Input: dimensioned drawing with shaded views. Units: mm. Origin: part minimum x, y, z. A direction names the side the tool comes from. Coordinates: 2 decimals unless noted, no trailing zeros. Order: outer loops, then holes, each group sorted by start corner. A loop starts at its lowest first (then second) coordinate and runs counter-clockwise, first axis right, second up.
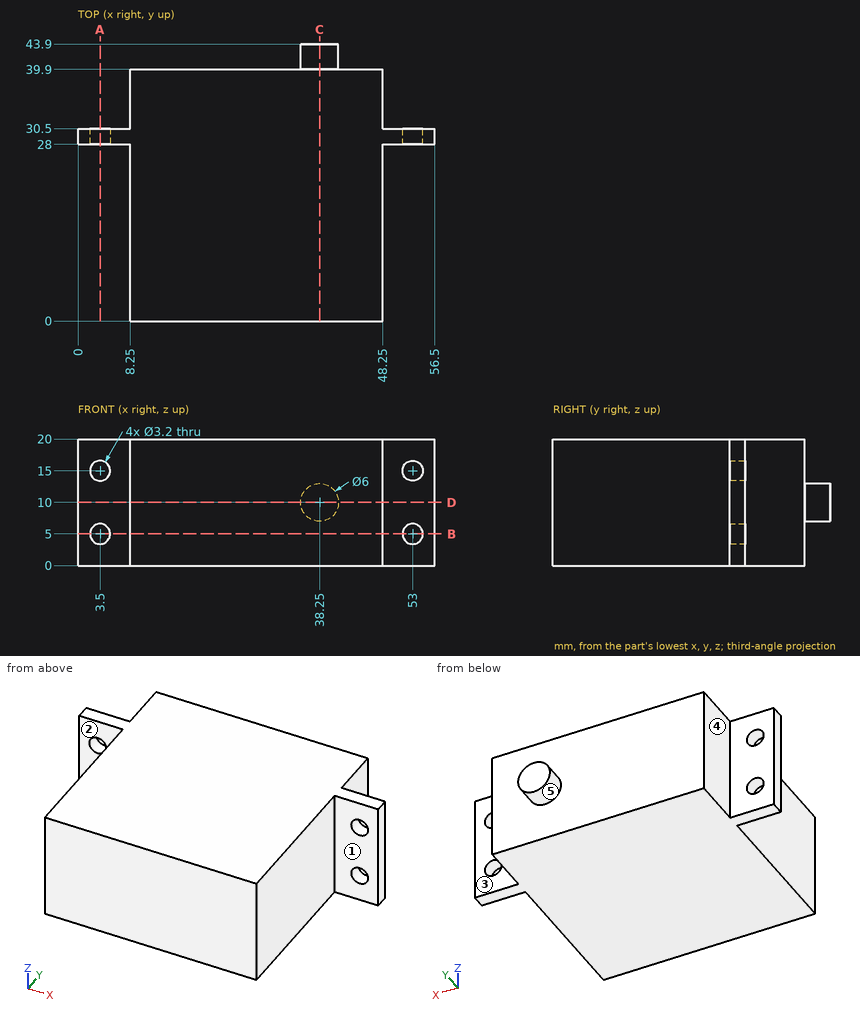
1. Section query D-D, the plane z = 10. Output: boundary loops of the cut face in (x, y), plus the area to 3 significant figures.
2. Contact query for flat-ended pins moving along their axis: P1, Ø5, axis at x = 45, z = 2.5, coming from the +Y side; P2, Ø7.5, axis at y = 36.5, z = 5.5, coming from the +X side; P3, Ø3.5, axis at x = 53, z = 15, coming from the -Y side. Output: stop coordinate, or through.
3. Section query C-C, the plane x = 38.25. Output: boundary loops of the cut face in (y, z), plus the area to 3 significant figures.
4. Section query A-A, the plane x = 3.5. Output: boundary loops of the cut face in (y, z), plus the area to 3 significant figures.
5. Section query B-B, the plane z = 5. Output: boundary loops of the cut face in (x, y), plus the area to 3 significant figures.
6. Material intervals for line 1 along X through (y, z) = (29, 15); line 2 along Z through (x, y) = (3.5, 28.65); line 3 along Z through (x, y) = (3, 29), sorted ascending.
7. Access query for the marked faces 1, 2, 3, 4 and 5. Directions: +Z, -Z, +X, -X, +Y, -Y. A direction counts if a zero-diameter tool reaches every point of the face in a straight line with its end or side. Return the directions, or none.
Answer key:
1. outline: (0, 28) - (8.25, 28) - (8.25, 0) - (48.25, 0) - (48.25, 28) - (56.5, 28) - (56.5, 30.5) - (48.25, 30.5) - (48.25, 39.9) - (41.25, 39.9) - (41.25, 43.9) - (35.25, 43.9) - (35.25, 39.9) - (8.25, 39.9) - (8.25, 30.5) - (0, 30.5) - close
1. area: 1,660 mm2
2. P1: stops at y = 39.9
2. P2: stops at x = 48.25
2. P3: stops at y = 28
3. outline: (0, 0) - (39.9, 0) - (39.9, 7) - (43.9, 7) - (43.9, 13) - (39.9, 13) - (39.9, 20) - (0, 20) - close
3. area: 822 mm2
4. outline: (28, 0) - (30.5, 0) - (30.5, 3.4) - (28, 3.4) - close; (28, 6.6) - (30.5, 6.6) - (30.5, 13.4) - (28, 13.4) - close; (28, 16.6) - (30.5, 16.6) - (30.5, 20) - (28, 20) - close
4. area: 34.0 mm2
5. outline: (0, 28) - (1.9, 28) - (1.9, 30.5) - (0, 30.5) - close; (5.1, 28) - (8.25, 28) - (8.25, 0) - (48.25, 0) - (48.25, 28) - (51.4, 28) - (51.4, 30.5) - (48.25, 30.5) - (48.25, 39.9) - (8.25, 39.9) - (8.25, 30.5) - (5.1, 30.5) - close; (54.6, 28) - (56.5, 28) - (56.5, 30.5) - (54.6, 30.5) - close
5. area: 1,620 mm2
6. line 1: x = 0 to 1.9, 5.1 to 51.4, 54.6 to 56.5
6. line 2: z = 0 to 3.4, 6.6 to 13.4, 16.6 to 20
6. line 3: z = 0 to 3.48, 6.52 to 13.48, 16.52 to 20
7. face 1: +Z, -Z, +X, -Y
7. face 2: +Z, -Z, -X, -Y
7. face 3: +Z, -Z, +X, +Y
7. face 4: +Z, -Z, -X, +Y
7. face 5: +Y
